Autodesk Fusion 360 part; units mm, degrees
sketch "Esboço1" plane through (0, 0, 0) normal (0, 0, 1) x (1, 0, 0)
  line L0 (13, 46.1) -> (21, 46.1)
  line L1 (13, 62.1) -> (13, 46.1)
  line L2 (-4, -4.1) -> (-4, 68.1)
  line L3 (-4, -4.1) -> (20.9993, -4.1)
  line L4 (21, 68.1) -> (21, 62.1)
  line L5 (21, 62.1) -> (13, 62.1)
  line L6 (20.9993, 3.9) -> (20.9993, -4.1)
  line L7 (21, 46.1) -> (21, 42.1)
  arc A0 (21, 42.1) -> (20.9993, 3.9) centre (21, 23) ccw
  line L8 (-4, 68.1) -> (21, 68.1)
  dimension "d2" = 16
  dimension "d3" = 8
  dimension "d5" = 6
  dimension "d8" = 8
  dimension "d10" = 8
  dimension "d36" = 25
  dimension "d12" = 4
  dimension "d13" = 19.1
extrude "Extrusão1" add sketch "Esboço1" along normal blind 30
hole "Furo1" at (-4, 65.1791, 15.483) direction (1, 0, 0) diameter 4 depth 25 tip angle 180
hole "Furo2" at (-4, 0.559, 14.816) direction (1, 0, 0) diameter 4 depth 25 tip angle 180
fillet "Arredondamento1" radius 1.5 5 edges at (-4, 32, 30) (-4, -4.1, 15) (8.4996, -4.1, 30) (8.4996, -4.1, 0) (-4, 32, 0)
fillet "Arredondamento2" radius 1.5 5 edges at (9.25, 68.1, 30) (-3.5607, 68.1, 29.5607) (-4, 68.1, 15) (-3.5607, 68.1, 0.4393) (9.25, 68.1, 0)
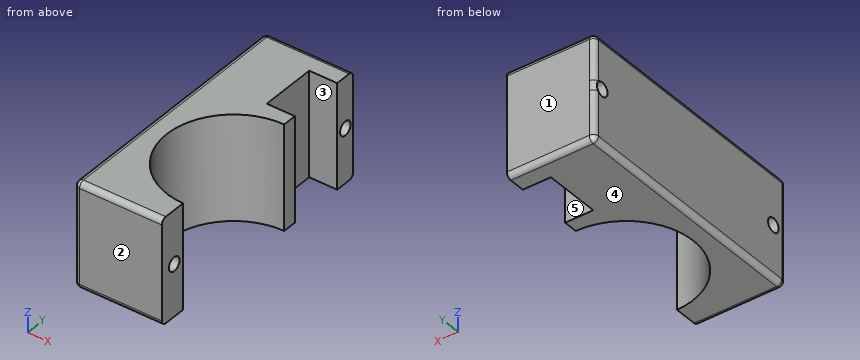
For this review, take the finished solid that the model builds, in its own axes (mm). Face numbers are marked on the shaded views. A direction names the side the tool comes from. Round coordinates to 2 decimals unless told otherwise and drop trailing zeros. Write each loop counter-clockwise with the first axis right and the second up, starting at its lowest first coordinate (ties: lowest second). Pieces come first, ordered by that corner, then holes. Notation, with made-up numbers: (23.25, -21) - (82.25, -21) arc R21 ccw to (82.25, 11) - close; hole circle Ø9 at (63, 22). An arc over 180 degrees is marked (long way). Write each question's results on one line, items separated by ' | '.
Item 1: Take a section at C-C on z = 20.75. State the section outline as (x, y) points, then the cut area to 3 significant figures.
Calculated:
outline: (-4, -2.6) arc R1.5 ccw to (-2.5, -4.1) - (21, -4.1) - (21, 3.9) arc R19.1 cw to (21, 42.1) - (21, 46.1) - (13, 46.1) - (13, 62.1) - (21, 62.1) - (21, 68.1) - (-2.5, 68.1) arc R1.5 ccw to (-4, 66.6) - close | area: 1,100 mm^2
Item 2: For pin 1 (5 mm diameter, centred on y = 49, z = 15, fed in from +X), flat-tipped, find the tip position at first contact; note if it passes through.
Calculated:
pin 1: stops at x = 13
Item 3: Take a section at D-D on x = 2.75. State the section outline as (y, z) points, then the cut area to 3 significant figures.
Calculated:
outline: (-4.1, 1.5) arc R1.5 ccw to (-2.6, 0) - (17.37, 0) - (17.37, 30) - (-2.6, 30) arc R1.5 ccw to (-4.1, 28.5) - close; (28.63, 0) - (66.6, 0) arc R1.5 ccw to (68.1, 1.5) - (68.1, 28.5) arc R1.5 ccw to (66.6, 30) - (28.63, 30) - close; hole circle Ø4 at (0.56, 14.82); hole circle Ø4 at (65.18, 15.48) | area: 1,800 mm^2
Item 4: Take a section at B-B on y = 23. State the section outline as (x, z) points.
Calculated:
outline: (-4, 1.5) arc R1.5 ccw to (-2.5, 0) - (1.9, 0) - (1.9, 30) - (-2.5, 30) arc R1.5 ccw to (-4, 28.5) - close
Item 5: Take a section at A-A on x = 6.75. State the section outline as (y, z) points, then the cut area to 3 significant figures.
Calculated:
outline: (-4.1, 1.5) arc R1.5 ccw to (-2.6, 0) - (10.28, 0) - (10.28, 30) - (-2.6, 30) arc R1.5 ccw to (-4.1, 28.5) - close; (35.72, 0) - (66.6, 0) arc R1.5 ccw to (68.1, 1.5) - (68.1, 28.5) arc R1.5 ccw to (66.6, 30) - (35.72, 30) - close; hole circle Ø4 at (0.56, 14.82); hole circle Ø4 at (65.18, 15.48) | area: 1,380 mm^2
Item 6: Draft analysis for pull direction Y (two halves, no side actions). For the marked faces 1, 2 and 3, state which applies: pulls with the +Y half, pulls with the -Y half, needs draft (parallel to the pull), parting line crosses it, or undercut.
Calculated:
face 1: pulls with the +Y half | face 2: pulls with the -Y half | face 3: undercut
Item 7: To check wall thickness, follow line 1 along Y through (x, z) = (18.5, 27.75); line 2 along Y through (x, z) = (5, 14.75); line 3 along Y through (x, z) = (19.25, 12.25). State the ranges of each line that lie inside material, in increasing order. Write a range as from..to.
Calculated:
line 1: y = -4.1..4.06, 41.94..46.1, 62.1..68.1 | line 2: y = -4.1..-1.44, 2.56..12.57, 33.43..63.32, 67.04..68.1 | line 3: y = -4.1..3.98, 42.02..46.1, 62.1..68.1
Item 8: For the marked faces 4 and 5, list the 3-axis set-ups (+Z, -Z, +X, -X, +Y, -Y) from which the entire face can be reached by the end or side of a thin tool; tool diameter is ignored.
Calculated:
face 4: -Z, +X, -X, +Y, -Y | face 5: +Z, -Z, +X
